Design review of the part built by this model. Coordinates are the model's own, in mm. Coordinates: 2 decimals unless noted, no trailing zeros. Order: outer loops, then holes, each group sorted by start corner. A loop starts at its lowest first (then second) coordinate and runs counter-clockwise, first axis right, second up. Notation, with made-up numbers: M 22.25,56.5 L 78.25,56.5 A28 ccw 78.25,78.5 Z; hole C -39,66 d10. An arc over 180 degrees is marked long. Answer as a JSON object with one key per item and string values.
from build123d import *

# Parameters (mm, degrees)
F0_W     = 101.6
F0_H     = 50.8
F1_DEPTH = 6.35
F2_R     = 1.65
F3_DEPTH = 25.4
F4_R     = 5.08


with BuildPart() as f1:
    # F0 (on Top) → F1 (new body)
    with BuildSketch(Plane.XY):
        Rectangle(F0_W, F0_H)
    extrude(amount=F1_DEPTH)

    # F2 (on face) → F3 (cut)
    with BuildSketch(Plane.XY.offset(6.35)):
        with Locations((-41.275, 10.885714)):
            Circle(F2_R)
        with Locations((-41.275, 3.628571)):
            Circle(F2_R)
        with Locations((-41.275, -3.628571)):
            Circle(F2_R)
        with Locations((-41.275, -10.885714)):
            Circle(F2_R)
        with Locations((-41.275, -18.142857)):
            Circle(F2_R)
        with Locations((-41.275, 18.142857)):
            Circle(F2_R)
        with Locations((41.275, 18.142857)):
            Circle(F2_R)
        with Locations((41.275, 10.885714)):
            Circle(F2_R)
        with Locations((41.275, 3.628571)):
            Circle(F2_R)
        with Locations((41.275, -3.628571)):
            Circle(F2_R)
        with Locations((41.275, -10.885714)):
            Circle(F2_R)
        with Locations((41.275, -18.142857)):
            Circle(F2_R)
    extrude(amount=-F3_DEPTH, mode=Mode.SUBTRACT)

    # F4
    f4_edges = [f1.edges().sort_by_distance(p)[0] for p in [
        (-50.8, 25.4, 3.175),
        (-50.8, -25.4, 3.175),
        (50.8, -25.4, 3.175),
        (50.8, 25.4, 3.175),
        (50.8, 0, 6.35),
        (0, 25.4, 6.35),
        (-50.8, 0, 6.35),
        (0, -25.4, 6.35),
    ]]
    fillet(f4_edges, radius=F4_R)


solid = f1.part
1) Add section B-B (x = -31.5). State the section outline as (y, z) points.
Taken from the geometry:
{"outline": "M -25.4,0 L 25.4,0 L 25.4,1.27 A5.08 ccw 20.32,6.35 L -20.32,6.35 A5.08 ccw -25.4,1.27 Z"}
2) Mouldability with a two-part tool opening along Y and no side actions: class faces 1 (the cylindrical face through (49.272, -23.951, 0.644)), 2 (the flat face through (-1, 0, 6.35)), 3 (the cylindrical face through (-42.923, -3.556, 3.219)), 4 (the cylindrical face through (49.272, 23.951, 0.644)) as released by +Y, released by -Y, zero draft, split by the parting line, or undercut.
Taken from the geometry:
{"face 1": "released by -Y", "face 2": "zero draft", "face 3": "undercut", "face 4": "released by +Y"}
3) Add section A-A (z = 2.25). Count the separate pieces of the cut face and the enclosed holes in it, and give its area (3 significant figures).
Taken from the geometry:
{"separate pieces": "1", "enclosed holes": "12", "area": "5,010 mm2"}
4) To check wall thickness, follow L1, parallel to X at y = 4, z = 3; L2, parallel to X at y = -4.5, z = 5.75 (3 decimals); L3, parallel to X at y = 14.5, z = 1.75. State the ranges of each line that lie inside material, in increasing order.
Taken from the geometry:
{"L1": "x = -50.5 to -42.88, -39.67 to 39.67, 42.88 to 50.5", "L2": "x = -48.115 to -42.676, -39.874 to 39.874, 42.676 to 48.115", "L3": "x = -50.78 to 50.78"}
5) Insertion check: pin 1 Ø2 at (x, z) = (-14, 3) entering from -Y; pin 2 Ø3 at (x, y) = (41.28, 18.14) entering from -Z. Each pin has a flat end and moves straight along its axis. Give the tip position at first contact, or say it passes through.
Taken from the geometry:
{"pin 1": "stops at y = -25.35", "pin 2": "passes through"}
6) Add section C-C (y = 6.5). State the section outline as (x, z) points.
Taken from the geometry:
{"outline": "M -50.8,0 L 50.8,0 L 50.8,1.27 A5.08 ccw 45.72,6.35 L -45.72,6.35 A5.08 ccw -50.8,1.27 Z"}
